Here's the drawing with two shaded views (mm, measured from the low corner). I have some questions. A direction names the side the tool comes from. Coordinates: 2 decimals unless noted, no trailing zeros. Write each loop counter-clockwise with the first axis right and the second up, starting at its lowest first coordinate (ties: lowest second). Pieces come first, ordered by that corner, then holes. Notation, with made-up numbers: M 5,37 L 49,37 A32 ccw 49,73 Z; hole C -23.75,24.5 d3. An arc over 180 degrees is marked long. Use one line per item in the form item = value. Start each with the question number.
1. I want a section at D-D, the plane z = 4. List the corners of the cut face in (x, y) for me.
2. I want a section at C-C, the plane z = 17.75. List the corners of the cut face in (x, y) for me, plus the area to 3 significant figures.
3. On a 3-axis mill with a long thin cutter (end or side, diameter ignored), from which of +Z, -Z, +X, -X, +Y, -Y can I reach the whole of each face in a straight line? I mean the marked faces 5, 6 and 7. Say none if no direction works.
4. Thinking about a two-plate mould opening in X: for the marked faces 1, 2, 3 and 4, which applies, released by +X, released by -X, zero draft, split by the parting line, or undercut?
5. Please list where these lines run through material, in increasing order: line 1 along X through (y, z) = (11, 12.75); line 2 along Y through (x, z) = (17, 4.5); line 3 along Y through (x, z) = (6.5, 4.5). Write a range as [from, to].
6. I want a section at A-A, the plane y = 11. List the corners of the cut face in (x, z) for me.
7. I'm going to push flat-ended pins straight in: pin 1 Ø5 at (y, z) = (9.5, 15.5) entering from +X; pin 2 Ø8 at (y, z) = (12.5, 16) entering from -X; pin 3 Ø3 at (x, z) = (10.5, 16) entering from +Y. Where does each tip first touch, or does it pass through?
8. I want a section at B-B, the plane x = 20. List the corners of the cut face in (y, z) for me.
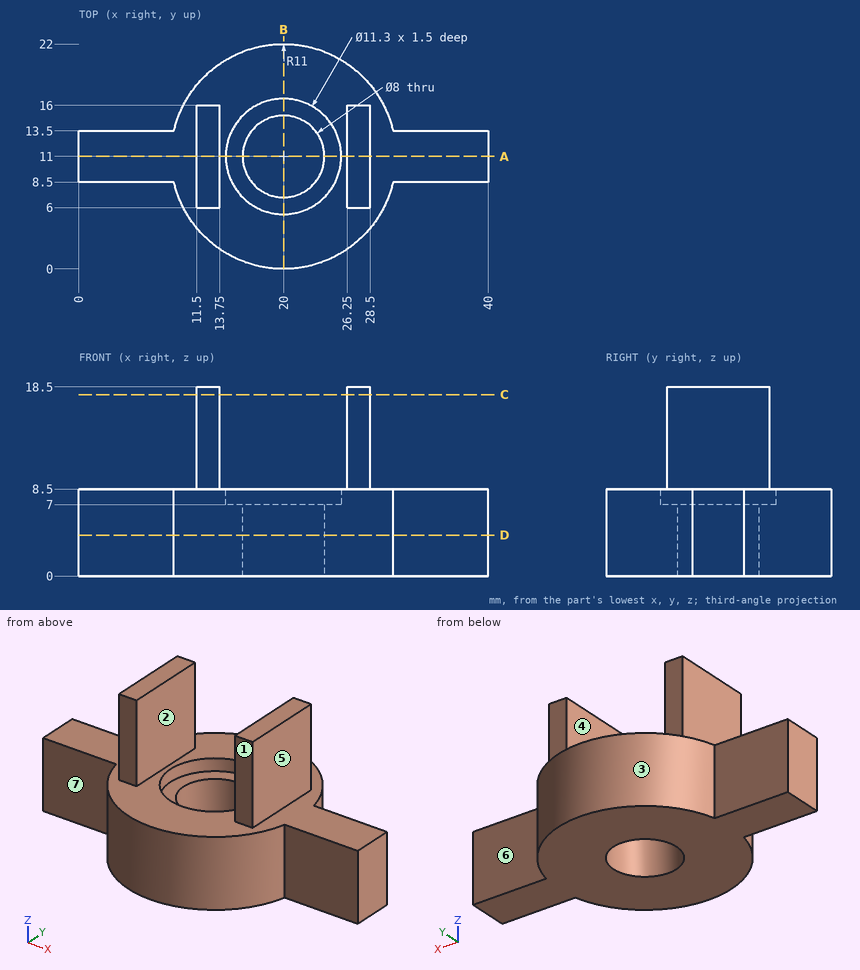
Answer list:
q1.outline = M 0,8.5 L 9.29,8.5 A11 ccw 30.71,8.5 L 40,8.5 L 40,13.5 L 30.71,13.5 A11 ccw 9.29,13.5 L 0,13.5 Z; hole C 20,11 d8
q2.outline = M 11.5,6 L 13.75,6 L 13.75,16 L 11.5,16 Z; M 26.25,6 L 28.5,6 L 28.5,16 L 26.25,16 Z
q2.area = 45.0 mm²
q3.face_5 = +Z, +X, +Y, -Y
q3.face_6 = +Z, -Z, +X, +Y
q3.face_7 = +Z, -Z, -X, -Y
q4.face_1 = zero draft
q4.face_2 = undercut
q4.face_3 = split by the parting line
q4.face_4 = undercut
q5.line_1 = [11.5, 13.75], [26.25, 28.5]
q5.line_2 = [0.42, 8.35], [13.65, 21.58]
q5.line_3 = [8.5, 13.5]
q6.outline = M 0,0 L 16,0 L 16,7 L 14.35,7 L 14.35,8.5 L 13.75,8.5 L 13.75,18.5 L 11.5,18.5 L 11.5,8.5 L 0,8.5 Z; M 24,0 L 40,0 L 40,8.5 L 28.5,8.5 L 28.5,18.5 L 26.25,18.5 L 26.25,8.5 L 25.65,8.5 L 25.65,7 L 24,7 Z
q7.pin_1 = 28.5
q7.pin_2 = 11.5
q7.pin_3 = 16
q8.outline = M 0,0 L 7,0 L 7,7 L 5.35,7 L 5.35,8.5 L 0,8.5 Z; M 15,0 L 22,0 L 22,8.5 L 16.65,8.5 L 16.65,7 L 15,7 Z
